from build123d import *

# Parameters (mm, degrees)
F0_W         = 2.3
F0_H         = 2
F0_W_2       = 2
F1_DEPTH     = 119.5
F2_T         = -2
F3_DEPTH     = 3.35
F4_DEPTH     = 2.5
F5_START     = -19
F5_DEPTH     = 16.5
F6_START     = -21.5
F6_DEPTH     = 11.65
F8_W         = 11.65
F8_H         = 1
F9_DEPTH     = 0.25
F10_T1_DEPTH = 42.6433659759
F10_T3_DEPTH = 8.6788998819
F10_T5_DEPTH = 121.7571417204
F11_R        = 5


# Not quite as in the source:
# - a fillet or chamfer that OpenCascade refuses, or shapes differently, is made with other operations: its cross-section is extruded or revolved along the edge and cut away or added
# - a pattern or mirror of a feature is missing from the dataset's text; its kind, count and spacing are read off the source's solid


with BuildPart() as f1:
    # F0 (on Right) → F1 (new body)
    with BuildSketch(Plane.YZ):
        with Locations((-17.4, 6)):
            Rectangle(F0_W, F0_H)
        Polygon((-21.25, 2.5), (-20, 1.25), (-16.25, 5), (-18.55, 5), (-18.55, 7), (-16.25, 7), (-16.25, 9), (-21.25, 9), align=None)
        Polygon((-18.75, 0), (18.75, 0), (18.75, 3), (16.75, 3), (16.75, 5), (-16.25, 5), (-20, 1.25), align=None)
        with Locations((17.75, 4)):
            Rectangle(F0_W_2, F0_H)
    extrude(amount=-F1_DEPTH)

    # F2
    f2_openings = [f1.faces().sort_by_distance(p)[0] for p in [
        (-59.75, 1.25, 5),
        (-59.75, -16.25, 7),
        (-59.75, -18.75, 9),
    ]]
    offset(amount=F2_T, openings=f2_openings)

    # F0 (on Right) → F3 (join)
    with BuildSketch(Plane.YZ):
        with Locations((-17.4, 6)):
            Rectangle(F0_W, F0_H)
        Polygon((-21.25, 2.5), (-20, 1.25), (-16.25, 5), (-18.55, 5), (-18.55, 7), (-16.25, 7), (-16.25, 9), (-21.25, 9), align=None)
    f3 = extrude(amount=-F3_DEPTH)

    # F3_copies: F3 across plane
    add(f3.mirror(Plane(origin=(-59.75, 0, 0), x_dir=(0, 0, -1), z_dir=(-1, 0, 0))))

    # F0 (on Right) → F4 (cut)
    with BuildSketch(Plane.YZ):
        with Locations((-17.4, 6)):
            Rectangle(F0_W, F0_H)
    f4 = extrude(amount=-F4_DEPTH, mode=Mode.SUBTRACT)

    # F4_copies: F4 across plane
    add(f4.mirror(Plane(origin=(-59.75, 0, 0), x_dir=(0, 0, -1), z_dir=(-1, 0, 0))), mode=Mode.SUBTRACT)

    # F0 (on Right) → F5 (cut)
    with BuildSketch(Plane.YZ.offset(F5_START)):
        with Locations((17.75, 4)):
            Rectangle(F0_W_2, F0_H)
    f5 = extrude(amount=-F5_DEPTH, mode=Mode.SUBTRACT)

    # F5_copies: F5 across plane
    add(f5.mirror(Plane(origin=(-59.75, 0, 0), x_dir=(0, 0, -1), z_dir=(-1, 0, 0))), mode=Mode.SUBTRACT)

    # F0 (on Right) → F6 (join)
    with BuildSketch(Plane.YZ.offset(F6_START)):
        with Locations((17.75, 4)):
            Rectangle(F0_W_2, F0_H)
        Polygon((16.75, 5), (18.75, 5), (20.75, 5), (20.75, 3.7), (20.95, 3.7), (22.25, 5), (22.25, 6.5), (16.75, 6.5), align=None)
    f6 = extrude(amount=-F6_DEPTH)

    # F6_copies: F6 across plane
    add(f6.mirror(Plane(origin=(-59.75, 0, 0), x_dir=(0, 0, -1), z_dir=(-1, 0, 0))))

    # F8 (on face) → F9 (cut)
    with BuildSketch(Plane(origin=(0, 0, 0), x_dir=(1, 0, 0), z_dir=(0, 0, -1))):
        with Locations((-27.325, -16.25)):
            Rectangle(F8_W, F8_H)
        with Locations((-27.325, -14.25)):
            Rectangle(F8_W, F8_H)
        with Locations((-27.325, -12.25)):
            Rectangle(F8_W, F8_H)
        with Locations((-27.325, -10.25)):
            Rectangle(F8_W, F8_H)
        with Locations((-27.325, -8.25)):
            Rectangle(F8_W, F8_H)
        with Locations((-27.325, -6.25)):
            Rectangle(F8_W, F8_H)
    f9 = extrude(amount=-F9_DEPTH, mode=Mode.SUBTRACT)

    # F9_copies: F9 across plane
    add(f9.mirror(Plane(origin=(-59.75, 0, 0), x_dir=(0, 0, -1), z_dir=(-1, 0, 0))), mode=Mode.SUBTRACT)

    # F10: chamfer of 1 on 5 edges, made by hand

    # F10_s2 → F10_t1 (cut)
    with BuildSketch(Plane.XZ.offset(-21.321682988)):
        Polygon((0, 1), (-1, 0), (0, 0), align=None)
        Polygon((-119.5, 1), (-118.5, 0), (-119.5, 0), align=None)
    extrude(amount=F10_T1_DEPTH, mode=Mode.SUBTRACT)

    # F10_s4 → F10_t3 (cut)
    with BuildSketch(Plane(origin=(0, -13.6934544799, 13.6934544799), x_dir=(1, 0, 0), z_dir=(0, 0.7071067812, -0.7071067812))):
        Polygon((0, 12.2582521472), (-1, 13.2582521472), (0, 13.2582521472), align=None)
        Polygon((-119.5, 12.2582521472), (-118.5, 13.2582521472), (-119.5, 13.2582521472), align=None)
    extrude(amount=F10_T3_DEPTH, mode=Mode.SUBTRACT)

    # F10_s6 → F10_t5 (cut)
    with BuildSketch(Plane.YZ.offset(-120.6285708602)):
        Polygon((-21.25, 2.9142135624), (-20.9571067812, 2.2071067812), (-21.25, 2.5), align=None)
    extrude(amount=F10_T5_DEPTH, mode=Mode.SUBTRACT)

    # F11
    f11_edges = [f1.edges().sort_by_distance(p)[0] for p in [
        (0, 18.75, 3),
        (-119.5, 18.75, 3),
        (-2, 16.75, 3.5),
        (-117.5, 16.75, 3.5),
    ]]
    fillet(f11_edges, radius=F11_R)


solid = f1.part
The listing builds one solid part. Answer for the finished solid, in the listing's coordinates (mm). A direction names the side the tool comes from. Give positions to 0.01 mm unless a question says otherwise; leave off trailing zeros. Write each loop counter-clockwise with the first axis right and the second up, starting at its lowest first coordinate (ties: lowest second). Pieces come first, ordered by that corner, then holes. Notation, with made-up numbers: (30, -27.75) -> (60, -27.75) arc R28 cw to (60, 6.25) -> close; hole circle Ø5 at (72.5, -11). An arc over 180 degrees is marked (long way). One line per question, with ' | ' between items. Start each with the question number.
1. Section A-A (x = -61.5) is taken. Determine the outline of the cut face in (y, z), plus the area to 3 significant figures.
2. For faces 5 (the flat face through (-59, 16.75, 4)), 6 (the flat face through (-116.83, -17.43, 3.82)), 7 (the flat face through (-100.5, 18, 4)), determine the directions among +Z, -Z, +X, -X, +Y, -Y from which every point of the face is accessible in a straight line to the end or side of a thin tool.
3. Find the intervals of material crossed by probe 1 along X at (y, z) = (-7, 4); probe 2 along Z at (x, y) = (-89, 6); probe 3 along X at (y, z) = (-18, 8.25), in increasing order.
4. For a pull along Z with two mould halves and no side action, classify faces 1 (the flat face through (-60, 18, 5)), 2 (the flat face through (-1, -17, 7)), 3 (the flat face through (-2.5, -17, 6)), 4 (the flat face through (-119.5, -4, 3)) as pulls with the +Z half, pulls with the -Z half, needs draft (parallel to the pull), parting line crosses it, or undercut.
5. Section B-B (y = -9) is taken. Determine the outline of the cut face in (x, z).
6. Given pin 1 Ø3 at (x, y) = (-100.5, -16.5) entering from +Z; pin 2 Ø5 at (x, z) = (-66, 5.5) entering from +Y; pin 3 Ø5 at (x, z) = (-93.5, 1.5) entering from +Y, each flat-ended and moving along its own axis, determine where each tip first touches the part or whether it passes through.
Response values:
1) outline: (-21.25, 2.91) -> (-20.96, 2.21) -> (-18.75, 0) -> (18.75, 0) -> (18.75, 5) -> (16.75, 5) -> (16.75, 2) -> (-17.92, 2) -> (-19.25, 3.33) -> (-19.25, 9) -> (-21.25, 9) -> close | area: 97.7 mm2
2) face 5: +Z | face 6: none | face 7: +Z, +Y
3) probe 1: -119.5 to -117.5, -2 to 0 | probe 2: 0.25 to 2 | probe 3: -119.5 to -116.15, -3.35 to 0
4) face 1: pulls with the +Z half | face 2: undercut | face 3: undercut | face 4: needs draft
5) outline: (-119.5, 1) -> (-118.5, 0) -> (-1, 0) -> (0, 1) -> (0, 5) -> (-2, 5) -> (-2, 2) -> (-117.5, 2) -> (-117.5, 5) -> (-119.5, 5) -> close
6) pin 1: z = 2.08 | pin 2: y = 18.75 | pin 3: y = 21.25
